For this review, take the finished solid that the model builds, in its own axes (mm). Face numbers are marked on the shaded views. A direction names the side the tool comes from. Round coordinates to 2 decimals unless told otherwise and drop trailing zeros. Loops run counter-clockwise (first coordinate to the right, second up) from the corner with the lowest first, then second, coordinate; pieces in that order, holes last. Notation, with made-up numbers: M -15.5,-29 L 37.5,-29 A18 cw 37.5,-4 Z; hole C -35.75,-18.75 d5. An arc over 180 degrees is marked long. One line per question, with ' | ' between items. Start each with the question number.
1) We need section A-A (z = -17). Give the boundary of the cut face in (x, y), and give its area (3 significant figures).
2) We need section D-D (y = 0.5). Give the boundary of the cut face in (x, z), and give its area (3 significant figures).
3) For pin 1 Ø5 at (x, y) = (4, -12.5) entering from +Z; pin 2 Ø3.5 at (x, y) = (5, -7) entering from -Z; pin 3 Ø5 at (x, z) = (8, 2.5) entering from -Y, all flat-tipped, find the tip position at first contact; note any pin that passes through.
4) For the marked faces 4, 5 and 6, list the 3-axis set-ups (+Z, -Z, +X, -X, +Y, -Y) from which the entire face can be reached by the end or side of a thin tool; tool diameter is ignored.
5) Mouldability with a two-part tool opening along Y and no side actions: class the marked faces 1, 2 and 3 as pulls with the +Y half, pulls with the -Y half, needs draft (parallel to the pull), parting line crosses it, or undercut.
6) We need section C-C (z = -2). Give the boundary of the cut face in (x, y).
7) We need section B-B (x = 8.5). Give the boundary of the cut face in (y, z), and give its area (3 significant figures).
8) For probe 1 along Y at (x, z) = (7.5, 1.5); probe 2 along Z at (x, y) = (6.75, 15.5); probe 3 along Z at (x, y) = (8.5, -1.5), list the stretches that pass through material, from the lowest coordinate up. Write a range as from..to.
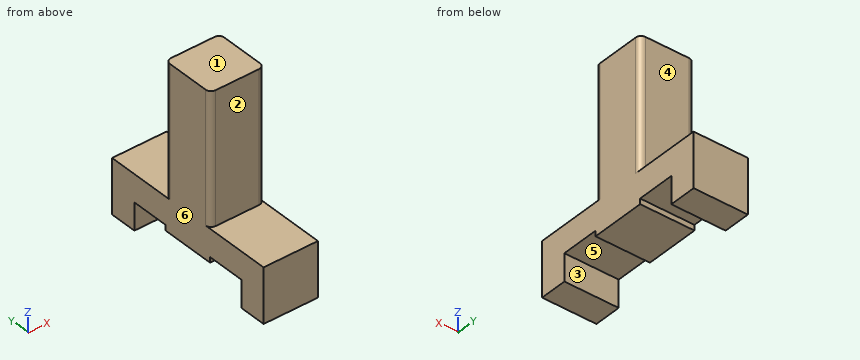
```python
from build123d import *

# Parameters (mm, degrees)
F0_W     = 10
F0_H     = 24
F0_H_2   = 5
F0_W_2   = 7
F0_W_3   = 5
F0_H_3   = 1
F1_DEPTH = 10
F2_R     = 1
F3_R     = 1
F4_R     = 1
F5_R     = 1


with BuildPart() as f1:
    # F0 (on Right) → F1 (new body)
    with BuildSketch(Plane.YZ):
        with Locations((0, 3)):
            Rectangle(F0_W, F0_H)
        with Locations((0, -11.5)):
            Rectangle(F0_W, F0_H_2)
        with Locations((8.5, -11.5)):
            Rectangle(F0_W_2, F0_H_2)
        with Locations((14.5, -11.5)):
            Rectangle(F0_W_3, F0_H_2)
        with Locations((14.5, -16.5)):
            Rectangle(F0_W_3, F0_H_2)
        with Locations((-8.5, -11.5)):
            Rectangle(F0_W_2, F0_H_2)
        with Locations((-14.5, -11.5)):
            Rectangle(F0_W_3, F0_H_2)
        with Locations((-14.5, -16.5)):
            Rectangle(F0_W_3, F0_H_2)
        with Locations((0, -14.5)):
            Rectangle(F0_W, F0_H_3)
    extrude(amount=F1_DEPTH)

    # F2
    f2_edges = [f1.edges().sort_by_distance(p)[0] for p in [
        (0, 5, 3),
    ]]
    fillet(f2_edges, radius=F2_R)

    # F3
    f3_edges = [f1.edges().sort_by_distance(p)[0] for p in [
        (10, 5, 3),
    ]]
    fillet(f3_edges, radius=F3_R)

    # F4
    f4_edges = [f1.edges().sort_by_distance(p)[0] for p in [
        (0, -5, 3),
    ]]
    fillet(f4_edges, radius=F4_R)

    # F5
    f5_edges = [f1.edges().sort_by_distance(p)[0] for p in [
        (10, -5, 3),
    ]]
    fillet(f5_edges, radius=F5_R)


solid = f1.part
```
Answers below:
1) outline: M 0,-17 L 10,-17 L 10,-12 L 0,-12 Z; M 0,12 L 10,12 L 10,17 L 0,17 Z | area: 100 mm^2
2) outline: M 0,-15 L 10,-15 L 10,15 L 0,15 Z | area: 300 mm^2
3) pin 1: z = -9 | pin 2: z = -14 | pin 3: y = -5
4) face 4: +Z, +X, -X, +Y | face 5: -Z, +X, -X | face 6: +Z, -Z, -X, +Y, -Y
5) face 1: needs draft | face 2: pulls with the -Y half | face 3: undercut
6) outline: M 0,-4 A1 ccw 1,-5 L 9,-5 A1 ccw 10,-4 L 10,4 A1 ccw 9,5 L 1,5 A1 ccw 0,4 Z
7) outline: M -17,-19 L -12,-19 L -12,-14 L -5,-14 L -5,-15 L 5,-15 L 5,-14 L 12,-14 L 12,-19 L 17,-19 L 17,-9 L 5,-9 L 5,15 L -5,15 L -5,-9 L -17,-9 Z | area: 470 mm^2
8) probe 1: -5..5 | probe 2: -19..-9 | probe 3: -15..15
